from build123d import *

# Parameters (mm, degrees)
SKETCH1_W           = 58
SKETCH1_H           = 32
BOSS_EXTRUDE1_DEPTH = 1.5
SKETCH1_3_W         = 9
SKETCH1_3_H         = 1.5
BOSS_EXTRUDE2_DEPTH = 23
SKETCH2_R           = 1.5
CUT_EXTRUDE1_DEPTH  = 49.928519291
SKETCH1_4_W         = 37
SKETCH1_4_H         = 1.5
BOSS_EXTRUDE3_DEPTH = 23
SKETCH3_R           = 2.5
CUT_EXTRUDE2_DEPTH  = 48.960921592
SKETCH1_5_R         = 2.5
CUT_EXTRUDE3_DEPTH  = 25


with BuildPart() as part:
    # Sketch1 → Boss-Extrude1 (new body)
    with BuildSketch(Plane(origin=(0, 0, 0), x_dir=(1, 0, 0), z_dir=(0, 1, 0))):
        Rectangle(SKETCH1_W, SKETCH1_H)
    extrude(amount=-BOSS_EXTRUDE1_DEPTH)

    # Sketch1_3 → Boss-Extrude2 (add)
    with BuildSketch(Plane(origin=(0, 0, 0), x_dir=(1, 0, 0), z_dir=(0, 1, 0))):
        with Locations((-24.5, -15.25)):
            Rectangle(SKETCH1_3_W, SKETCH1_3_H)
        with Locations((24.5, -15.25)):
            Rectangle(SKETCH1_3_W, SKETCH1_3_H)
    extrude(amount=BOSS_EXTRUDE2_DEPTH)

    # Sketch2 → Cut-Extrude1 (cut, through all)
    with BuildSketch(Plane.XY.offset(16)):
        with Locations((-23.5, 19.197487824)):
            Circle(SKETCH2_R)
        with Locations((-23.5, 8.197487824)):
            Circle(SKETCH2_R)
        with Locations((23.5, 17.446590768)):
            Circle(SKETCH2_R)
        with Locations((23.5, 8.197487824)):
            Circle(SKETCH2_R)
    extrude(amount=-CUT_EXTRUDE1_DEPTH, mode=Mode.SUBTRACT)

    # Sketch1_4 → Boss-Extrude3 (add)
    with BuildSketch(Plane(origin=(0, 0, 0), x_dir=(1, 0, 0), z_dir=(0, 1, 0))):
        with Locations((0, 15.25)):
            Rectangle(SKETCH1_4_W, SKETCH1_4_H)
    extrude(amount=BOSS_EXTRUDE3_DEPTH)

    # Sketch3 → Cut-Extrude2 (cut, through all)
    with BuildSketch(Plane.XY.offset(-14.5)):
        with Locations((10, 12.822039296)):
            Circle(SKETCH3_R)
        with Locations((-10, 12.822039296)):
            Circle(SKETCH3_R)
    extrude(amount=-CUT_EXTRUDE2_DEPTH, mode=Mode.SUBTRACT)

    # Sketch1_5 → Cut-Extrude3 (cut)
    with BuildSketch(Plane(origin=(0, 0, 0), x_dir=(1, 0, 0), z_dir=(0, 1, 0))):
        with Locations(Location((20, 0, 0), (0, 0, 270))):
            Circle(SKETCH1_5_R)
        with Locations(Location((0, 0, 0), (0, 0, 270))):
            Circle(SKETCH1_5_R)
        with Locations(Location((-20, 0, 0), (0, 0, 270))):
            Circle(SKETCH1_5_R)
    extrude(amount=-CUT_EXTRUDE3_DEPTH, mode=Mode.SUBTRACT)


solid = part.part
Can you work these out from the model? Positions are in its coordinate system, mm. A direction names the side the tool comes from. Give positions to 0.01 mm unless a question says otherwise; leave off trailing zeros. Write each loop counter-clockwise with the first axis right and the second up, starting at its lowest first coordinate (ties: lowest second). Pieces come first, ordered by that corner, then holes. Notation, with made-up numbers: M 12.25,85 L 28.25,85 A5 cw 28.25,92 Z; hole C 60,88 d5. An arc over 180 degrees is marked long. Answer in a Markdown table with one row per item. Add a question column.
Item 1: Please list where these lines run through material, in increasing order: L1, parallel to X at y = -0.6, z = 0; L2, parallel to Y at x = -23.5, z = 15.55; L3, parallel to X at y = 4.5, z = 15.
Item 2: For pin 1 Ø10 at (x, y) = (26, 14) entering from -Z; pin 2 Ø12 at (x, z) = (-11.5, -1.5) entering from +Y; pin 3 Ø1.2 at (y, z) = (6.5, -15.5) entering from +X, each with a flat end and sliding along its axis, tell me the tip position at first contact or that it passes through.
Item 3: Imagine slicing it at A-A, the plane x = -23.5. Write out the boundary of the cut face in (y, z).
Item 4: On a 3-axis mill with a long thin cutter (end or side, diameter ignored), from which of +Z, -Z, +X, -X, +Y, -Y can I reach the whole of each face in a straight line? I mean faces 1 (the flat face through (-25, 11, 14.5)), 2 (the flat face through (18.5, 11, -15)), 3 (the flat face through (-18.5, 11, -15)), 4 (the flat face through (20, 11, 15)). Say none if no direction works.
Item 5: Imagine slicing it at D-D, the plane x = 21. Write out the boundary of the cut face in (y, z).
Item 6: We'd pull the mould along Y, two halves only. Please class faces 5 (the cylindrical face through (-11.984, 11.301, -15.24)), 6 (the flat face through (24, 11, 14.5)), 7 (the flat face through (0, -1.5, -4)): released by +Y, released by -Y, zero draft, split by the parting line, or undercut.
Item 7: Imagine slicing it at C-C, the plane y = 1. Write out the boundary of the cut face in (x, z), plus the area to 3 significant figures.
Item 8: Imagine slicing it at B-B, the plane z = 0. Write out the boundary of the cut face in (x, y).
Evaluation:
| question | item | result |
|---|---|---|
| 1 | L1 | x = -29 to -22.5, -17.5 to -2.5, 2.5 to 17.5, 22.5 to 29 |
| 1 | L2 | y = -1.5 to 6.7, 9.7 to 17.7, 20.7 to 23 |
| 1 | L3 | x = -29 to -20, 20 to 29 |
| 2 | pin 1 | stops at z = 14.5 |
| 2 | pin 2 | stops at y = 0 |
| 2 | pin 3 | stops at x = 18.5 |
| 3 | outline | M -1.5,-16 L 0,-16 L 0,14.5 L 6.7,14.5 L 6.7,16 L -1.5,16 Z; M 9.7,14.5 L 17.7,14.5 L 17.7,16 L 9.7,16 Z; M 20.7,14.5 L 23,14.5 L 23,16 L 20.7,16 Z |
| 4 | face 1 | -Z, +X, -X, +Y |
| 4 | face 2 | +Z, -Z, +X, +Y |
| 4 | face 3 | +Z, -Z, -X, +Y |
| 4 | face 4 | +Z, -Z, +Y |
| 5 | outline | M -1.5,-16 L 0,-16 L 0,-2.29 L -1.5,-2.29 Z; M -1.5,2.29 L 0,2.29 L 0,14.5 L 23,14.5 L 23,16 L -1.5,16 Z |
| 6 | face 5 | undercut |
| 6 | face 6 | zero draft |
| 6 | face 7 | released by -Y |
| 7 | outline | M -29,14.5 L -20,14.5 L -20,16 L -29,16 Z; M -18.5,-16 L 18.5,-16 L 18.5,-14.5 L -18.5,-14.5 Z; M 20,14.5 L 29,14.5 L 29,16 L 20,16 Z |
| 7 | area | 82.5 mm² |
| 8 | outline | M -29,-1.5 L -22.5,-1.5 L -22.5,0 L -29,0 Z; M -17.5,-1.5 L -2.5,-1.5 L -2.5,0 L -17.5,0 Z; M 2.5,-1.5 L 17.5,-1.5 L 17.5,0 L 2.5,0 Z; M 22.5,-1.5 L 29,-1.5 L 29,0 L 22.5,0 Z |
